The listing builds one solid part. Answer for the finished solid, in the listing's coordinates (mm). Face numbers are marked on the shaded views. Give positions to 0.01 mm unless a question says otherwise; leave off trailing zeros. Order: outer loops, then holes, each group sorted by start corner. A loop starts at its lowest first (then second) coordinate and runs counter-clockwise, first axis right, second up. Notation, with made-up numbers: (41.25, -39.75) - (55.25, -39.75) arc R29 ccw to (55.25, -15.75) - close; hole circle Ø5 at (85.5, 64.5). An arc over 180 degrees is marked (long way). Write each question's results on one line, items separated by ' | '. Start each with the question number.
1. Section D-D (x = -7) is taken. Give the vertices of the cut face in (y, z) (3 decimals), and give its area (3 significant figures).
2. Find the intervals of material crossed by L1, parallel to X at y = 0, z = 0.05; L2, parallel to Z at x = -12, y = 17.5 (3 decimals); L3, parallel to X at y = -16.5, z = 9.25, in increasing order.
3. Section B-B (z = 7.75) is taken. Give the vertices of the cut face in (x, y), and give its area (3 significant figures).
4. Section A-A (y = 0) is taken. State how many separate pieces and enclosed holes the cut face has, and give its area (3 significant figures).
5. Section C-C (y = -8) is taken. Give the vertices of the cut face in (x, z) (3 decimals), and give its area (3 significant figures).
6. Flat-ended cylindrical pins translate along their axes: pin 1 (1 mm diameter, centred on y = 17.5, z = 0.5, fed in from +X); pin 2 (6 mm diameter, centred on x = 21.19, y = 0, fed in from +Z) (3 decimals); pin 3 (1 mm diameter, centred on x = -22.5, z = 0, fed in from -Y). Find the tip coordinate at first contact, or state that the pin passes through.
7. Determine the mould class of the marked faces 1, 2 and 3 for opening direction Z: released by +Z, released by -Z, zero draft, split by the parting line, or undercut.
from build123d import *

# Parameters (mm, degrees)
F1_DEPTH    = 25.4
F2_T1_DEPTH = 55.3405811878
F2_T3_DEPTH = 54.61
F2_T5_DEPTH = 51.133331808
F3_R        = 2.2479
F4_DEPTH    = 1.27


# Not quite as in the source:
# - a fillet or chamfer that OpenCascade refuses, or shapes differently, is made with other operations: its cross-section is extruded or revolved along the edge and cut away or added


with BuildPart() as f1:
    # F0 (on Front) → F1 (new body, symmetric)
    with BuildSketch(Plane.XZ):
        Polygon((-14.4773686111, 15.875), (-17.1645917971, 0.635), (-15.875, 0.635), (-12.9638415485, 17.145), (-16.7738415485, 17.145), (-16.7738415485, 15.875), align=None)
        Polygon((-15.875, 0.635), (-17.1645917971, 0.635), (-17.1645917971, -0.635), (17.1645917971, -0.635), (17.1645917971, 0.635), (15.875, 0.635), align=None)
        Polygon((12.9638415485, 17.145), (15.875, 0.635), (17.1645917971, 0.635), (14.4773686111, 15.875), (16.7738415485, 15.875), (16.7738415485, 17.145), align=None)
    extrude(amount=F1_DEPTH, both=True)

    # F2: fillet of radius 0.762 on 8 edges, made by hand

    # F2_s2 → F2_t1 (cut)
    with BuildSketch(Plane.XZ.offset(-27.6702905939)):
        with BuildLine():
            ThreePointArc((-13.8719577861, 17.145), (-13.2882319204, 16.8728041586), (-13.1215342783, 16.2506800886))
            Line((-13.1215342783, 16.2506800886), (-12.9638415485, 17.145))
            Line((-12.9638415485, 17.145), (-13.8719577861, 17.145))
        make_face()
        with BuildLine():
            ThreePointArc((13.1215342783, 16.2506800886), (13.2882319204, 16.8728041586), (13.8719577861, 17.145))
            Line((13.8719577861, 17.145), (12.9638415485, 17.145))
            Line((12.9638415485, 17.145), (13.1215342783, 16.2506800886))
        make_face()
    extrude(amount=F2_T1_DEPTH, mode=Mode.SUBTRACT)

    # F2_s4 → F2_t3 (cut)
    with BuildSketch(Plane.XZ.offset(-27.305)):
        with BuildLine():
            ThreePointArc((-16.7738415485, 16.383), (-16.5506569158, 16.9218153673), (-16.0118415485, 17.145))
            Line((-16.0118415485, 17.145), (-16.7738415485, 17.145))
            Line((-16.7738415485, 17.145), (-16.7738415485, 16.383))
        make_face()
        with BuildLine():
            ThreePointArc((16.0118415485, 17.145), (16.5506569158, 16.9218153673), (16.7738415485, 16.383))
            Line((16.7738415485, 16.383), (16.7738415485, 17.145))
            Line((16.7738415485, 17.145), (16.0118415485, 17.145))
        make_face()
        with BuildLine():
            ThreePointArc((-16.0118415485, 15.875), (-16.5506569158, 16.0981846327), (-16.7738415485, 16.637))
            Line((-16.7738415485, 16.637), (-16.7738415485, 15.875))
            Line((-16.7738415485, 15.875), (-16.0118415485, 15.875))
        make_face()
        with BuildLine():
            ThreePointArc((16.7738415485, 16.637), (16.5506569158, 16.0981846327), (16.0118415485, 15.875))
            Line((16.0118415485, 15.875), (16.7738415485, 15.875))
            Line((16.7738415485, 15.875), (16.7738415485, 16.637))
        make_face()
    extrude(amount=F2_T3_DEPTH, mode=Mode.SUBTRACT)

    # F2_s6 → F2_t5 (cut)
    with BuildSketch(Plane.XZ.offset(-25.566665904)):
        with BuildLine():
            ThreePointArc((-17.1530153049, 0.7006535498), (-17.161692157, 0.6347463144), (-17.1645917971, 0.5683336384))
            Line((-17.1645917971, 0.5683336384), (-17.1645917971, 0.635))
            Line((-17.1645917971, 0.635), (-17.1530153049, 0.7006535498))
        make_face()
        with BuildLine():
            ThreePointArc((17.1530153049, 0.7006535498), (17.161692157, 0.6347463144), (17.1645917971, 0.5683336384))
            Line((17.1645917971, 0.5683336384), (17.1645917971, 0.635))
            Line((17.1645917971, 0.635), (17.1530153049, 0.7006535498))
        make_face()
    extrude(amount=F2_T5_DEPTH, mode=Mode.SUBTRACT)

    # F3 (on face) → F4 (join)
    with BuildSketch(Plane(origin=(0, 0, -0.635), x_dir=(1, 0, 0), z_dir=(0, 0, -1))):
        with BuildLine():
            Line((-17.1645917971, 3.7719), (-17.1645917971, 5.0419))
            ThreePointArc((-17.1645917971, 5.0419), (-17.536566185, 4.1438743879), (-18.4345917971, 3.7719))
            Line((-18.4345917971, 3.7719), (-23.9463917971, 3.7719))
            ThreePointArc((-23.9463917971, 3.7719), (-24.8444174092, 3.3999256121), (-25.2163917971, 2.5019))
            Line((-25.2163917971, 2.5019), (-25.2163917971, -2.5019))
            ThreePointArc((-25.2163917971, -2.5019), (-24.8444174092, -3.3999256121), (-23.9463917971, -3.7719))
            Line((-23.9463917971, -3.7719), (-18.4345917971, -3.7719))
            ThreePointArc((-18.4345917971, -3.7719), (-17.536566185, -4.1438743879), (-17.1645917971, -5.0419))
            Line((-17.1645917971, -5.0419), (-17.1645917971, -3.7719))
            Line((-17.1645917971, -3.7719), (-17.1645917971, 3.7719))
        make_face()
        with Locations((-21.1904917971, 0)):
            Circle(F3_R, mode=Mode.SUBTRACT)
        with BuildLine():
            Line((23.9463917971, 3.7719), (18.4345917971, 3.7719))
            ThreePointArc((18.4345917971, 3.7719), (17.536566185, 4.1438743879), (17.1645917971, 5.0419))
            Line((17.1645917971, 5.0419), (17.1645917971, 3.7719))
            Line((17.1645917971, 3.7719), (17.1645917971, -3.7719))
            Line((17.1645917971, -3.7719), (17.1645917971, -5.0419))
            ThreePointArc((17.1645917971, -5.0419), (17.536566185, -4.1438743879), (18.4345917971, -3.7719))
            Line((18.4345917971, -3.7719), (23.9463917971, -3.7719))
            ThreePointArc((23.9463917971, -3.7719), (24.8444174092, -3.3999256121), (25.2163917971, -2.5019))
            Line((25.2163917971, -2.5019), (25.2163917971, 2.5019))
            ThreePointArc((25.2163917971, 2.5019), (24.8444174092, 3.3999256121), (23.9463917971, 3.7719))
        make_face()
        with Locations((21.1904917971, 0)):
            Circle(F3_R, mode=Mode.SUBTRACT)
    extrude(amount=-F4_DEPTH)


solid = f1.part
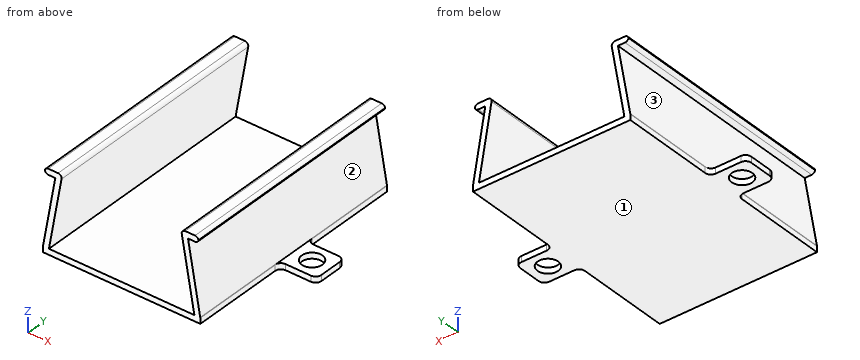
Reported:
1) outline: (-25.4, -0.635) - (25.4, -0.635) - (25.4, 0.635) - (-25.4, 0.635) - close | area: 64.5 mm²
2) L1: -25.22 to -23.44, -18.94 to 18.94, 23.44 to 25.22 | L2: -0.635 to 0.635 | L3: -15.65 to -14.36, 14.36 to 15.65
3) outline: (-15.91, -25.4) - (-14.62, -25.4) - (-14.62, 25.4) - (-15.91, 25.4) - close; (14.62, -25.4) - (15.91, -25.4) - (15.91, 25.4) - (14.62, 25.4) - close | area: 131 mm²
4) separate pieces: 3 | enclosed holes: 0 | area: 100 mm²
5) outline: (-17.165, -0.635) - (17.165, -0.635) - (17.165, 0.568) arc R0.762 ccw to (17.153, 0.701) - (14.477, 15.875) - (16.012, 15.875) arc R0.762 ccw to (16.763, 16.51) arc R0.762 ccw to (16.012, 17.145) - (13.872, 17.145) arc R0.762 ccw to (13.122, 16.251) - (15.875, 0.635) - (-15.875, 0.635) - (-13.122, 16.251) arc R0.762 ccw to (-13.872, 17.145) - (-16.012, 17.145) arc R0.762 ccw to (-16.763, 16.51) arc R0.762 ccw to (-16.012, 15.875) - (-14.477, 15.875) - (-17.153, 0.701) arc R0.762 ccw to (-17.165, 0.568) - close | area: 91.4 mm²
6) pin 1: x = 17.16 | pin 2: z = 0.635 | pin 3: y = -3.77
7) face 1: released by -Z | face 2: undercut | face 3: undercut
